Autodesk Inventor part; units mm, degrees
ref_plane "YZ Plane" through (0, 0, 0) normal (1, 0, 0) x (0, 1, 0)
ref_plane "XZ Plane" through (0, 0, 0) normal (0, 1, 0) x (-1, 0, 0)
ref_plane "XY Plane" through (0, 0, 0) normal (0, 0, 1) x (1, 0, 0)
sketch "Эскиз1" plane through (0, 0, 0) normal (0, 1, 0) x (-1, 0, 0)
  line L0 (0, -6.5) -> (-2.25, -6.5)
  line L1 (-2.25, -6.5) -> (-4.25, -6.5)
  line L2 (-2.25, -6.5) -> (-4.25, -6.5)
  line L3 (-6.5, -6.5) -> (-4.25, -6.5)
  line L4 (0, -6.5) -> (0, 0.5)
  line L5 (0, 0.5) -> (-6.5, 0.5)
  line L6 (-6.5, 0.5) -> (-6.5, -6.5)
  line L7 (-2.25, -6.5) -> (-2.25, -1.5)
  line L8 (-2.25, -1.5) -> (-4.25, -1.5)
  line L9 (-4.25, -1.5) -> (-4.25, -6.5)
  point P0 (0, 0)
  dimension "d2" = 2.25
  dimension "d4" = 2
  dimension "d31" = 7
  dimension "d32" = 5
extrude "Выдавливание1" add sketch "Эскиз1" along normal blind 21
sketch "Эскиз2" plane through (0, 21, 0) normal (0, 1, 0) x (1, 0, 0)
  line L0 (4.25, 2) -> (2.25, 2)
  line L1 (4.25, 6.5) -> (2.25, 6.5)
  line L2 (2.25, 6.5) -> (2.25, 2)
  line L3 (2.25, 2) -> (4.25, 2)
  line L4 (4.25, 2) -> (4.25, 6.5)
  point P0 (0, 0)
extrude "Выдавливание2" add sketch "Эскиз2" along normal blind 1.425 and the other way blind 22.425
sketch "Эскиз4" plane through (2.25, 0, -2) normal (0, 0, 1) x (1, 0, 0)
  line L0 (0, 22.425) -> (2, 22.425)
  line L1 (2, -1.425) -> (0, -1.425)
  line L2 (-2.25, 21) -> (4.75, 21)
  line L3 (-2.25, 0) -> (4.75, 0)
  line L4 (4.75, 0) -> (4.75, 21)
  line L5 (-2.25, 1) -> (-2.25, 20)
  line L6 (0, 22.425) -> (0, 21)
  line L7 (2, 21) -> (2, 22.425)
  dimension "d17" = 23.85
  dimension "d18" = 21
  dimension "d19" = 7
  dimension "d20" = 2.25
  dimension "d21" = 2
  dimension "d22" = 2.75
  dimension "d23" = 1.425
  dimension "d24" = 7
sketch "Эскиз6" plane through (0, 0, 0.5) normal (0, 0, 1) x (1, 0, 0)
  line L0 (0, 0) -> (0, 1.5)
  line L1 (0, 0) -> (0, 21)
  line L2 (0, 21) -> (6.5, 21)
  line L3 (0, 21) -> (0, 19.5)
  line L4 (0, 19.5) -> (5, 19.5)
  line L5 (5, 19.5) -> (5, 1.5)
  line L6 (5, 1.5) -> (0, 1.5)
  line L7 (0, 1.5) -> (0, 19.5)
  dimension "d33" = 1.5
  dimension "d34" = 1.5
  dimension "d35" = 5
extrude "Выдавливание5" cut sketch "Эскиз6" against normal blind 5
sketch "Эскиз7" plane through (6.5, 0, 0.5) normal (1, 0, 0) x (0, 0, -1)
  line L0 (7, 0) -> (7, 21)
  line L1 (7, 10.5) -> (7, 18)
  line L2 (7, 18) -> (7, 3)
  line L3 (0, 19.5) -> (0, 1.5)
  line L4 (0, 3) -> (7, 3)
  line L5 (0, 18) -> (7, 18)
  line L6 (7, 18) -> (4, 18)
  line L7 (4.5, 18) -> (4.5, 3)
  line L8 (4.5, 3) -> (2, 3)
  circle A0 centre (2, 3) radius 1.25
  circle A1 centre (4.25, 18) radius 1.25
  line L9 (5, 19.5) -> (5, 1.5)
  line L10 (5, 1.5) -> (5, 19.5)
  line L11 (5, 3) -> (5, 5)
  line L12 (5, 5) -> (5, 7)
  line L13 (5, 7) -> (5, 9)
  line L14 (5, 9) -> (5, 11)
  line L15 (5, 11) -> (5, 13)
  line L16 (5, 13) -> (5, 15)
  circle A2 centre (5, 5) radius 0.6
  circle A3 centre (5, 7) radius 0.6
  circle A4 centre (5, 9) radius 0.6
  circle A5 centre (5, 11) radius 0.6
  circle A6 centre (5, 13) radius 0.6
  circle A7 centre (5, 15) radius 0.6
  point P0 (0.5, 0)
  dimension "d38" = 7.5
  dimension "d39" = 15
  dimension "d40" = 3
  dimension "d41" = 0.5
  dimension "d42" = 2.5
  dimension "d43" = 2.5
  dimension "d44" = 2.5
  dimension "d61" = 2
  dimension "d62" = 2
  dimension "d63" = 2
  dimension "d64" = 2
  dimension "d65" = 2
  dimension "d66" = 2
  dimension "d68" = 1.2
  dimension "d69" = 1.2
  dimension "d70" = 1.2
  dimension "d71" = 1.2
  dimension "d72" = 1.2
  dimension "d73" = 1.2
extrude "Выдавливание6" add sketch "Эскиз7" along normal blind 1.7 contours A2 L7 L9 | L9 A2 | A1 L9 L5 | L5 L9 A1 | A0 L4 | L4 A0 | A2 L7 | L9 A1 L7 L5 | L5 A1 L9 | L7 A1 L5 | A7 L9 | L9 A7 L7 | A3 L7 | L7 A3 L9 | L9 A3 | L7 A7 | A4 L7 | L7 A4 L9 | A6 L9 L7 | L7 A6 | A6 L9 | L9 A4 | A5 L7 | L7 A5 L9 | L9 A5
properties part number "fast_battery"
The listing builds one solid part. Answer for the finished solid, in the listing's coordinates (mm). A direction names the side the tool comes from. Coordinates: 2 decimals unless noted, no trailing zeros. Loops run counter-clockwise (first coordinate to the right, second up) from the corner with the lowest first, then second, coordinate; pieces in that order, holes last. Notation, with made-up numbers: M 37,24.25 L 46,24.25 A21 ccw 46,56.25 Z; hole C 35.25,6.5 d5. An arc over 180 degrees is marked long. Answer as a JSON object with one key per item and string values. Group by question number.
Item 1: Consider L1, parallel to Y at x = 4, z = -3.5 (3 decimals); L2, parallel to Y at x = 1.5, z = -0.75; L3, parallel to X at y = 10.5, z = -3. Determine where each line is inside the solid, lowest interval first.
Item 2: Which of the six approach directions +Z, -Z, +X, -X, +Y, -Y give full straight-line access (tool end or side, diameter ignored) to faces 4 (the face through (3, -1, -2)), 5 (the face through (7.34, 14.59, -4.06)), 6 (the face through (4.25, 22, -4))?
Item 3: Each of these flat-tipped pins is pushed along its axis until it touches: P1, Ø1.1, axis at x = 3, y = 22, coming from the +Z side; P2, Ø1.5, axis at x = 6, z = -2, coming from the -Y side; P3, Ø0.7, axis at y = -1, z = -5, coming from the +X side. Where does it stop, or does it pass through?
Item 4: Determine the mould class of faces 1 (the face through (3, -1.425, -4)), 2 (the face through (7.338, 11.586, -4.37)), 3 (the face through (8.2, 9, -4.5)) for opening direction Y: +Y half, -Y half, draft (parallel to the pull), parting line (faces both ways), or undercut.
Item 5: Section C-C (z = -1.5) is taken. Write down the section's boundary in (x, y), and give its area (4 significant figures).
Item 6: Section B-B (y = 15) is taken. Write down the section's boundary in (x, z), and give its area (3 significant figures).
Item 7: Section D-D (y = 8) is taken. Write down the section's boundary in (x, z).
Item 8: Section A-A (x = 3.5) is taken. Write down the section's boundary in (y, z) (3 decimals), and give its area (3 significant figures).
Solved:
{
 "1": {"L1": "y = -1.425 to 1.5, 19.5 to 22.425", "L2": "y = 0 to 1.5, 19.5 to 21", "L3": "x = 5 to 6.5"},
 "2": {"face 4": "+Z, +X, -X, -Y", "face 5": "+X", "face 6": "+Z, -Z, +X, +Y"},
 "3": {"P1": "stops at z = -2", "P2": "stops at y = 0", "P3": "stops at x = 4.25"},
 "4": {"face 1": "-Y half", "face 2": "undercut", "face 3": "draft"},
 "5": {"outline": "M 0,0 L 6.5,0 L 6.5,1.75 L 8.2,1.75 L 8.2,4.25 L 6.5,4.25 L 6.5,21 L 0,21 L 0,19.5 L 5,19.5 L 5,1.5 L 0,1.5 Z", "area": "50.75 mm2"},
 "6": {"outline": "M 0,-6.5 L 6.5,-6.5 L 6.5,-5.1 L 8.2,-5.1 L 8.2,-3.9 L 6.5,-3.9 L 6.5,0.5 L 5,0.5 L 5,-4.5 L 0,-4.5 Z", "area": "22.5 mm2"},
 "7": {"outline": "M 0,-6.5 L 6.5,-6.5 L 6.5,0.5 L 5,0.5 L 5,-4.5 L 0,-4.5 Z"},
 "8": {"outline": "M -1.425,-6.5 L 22.425,-6.5 L 22.425,-2 L 21,-2 L 21,0.5 L 19.5,0.5 L 19.5,-4.5 L 1.5,-4.5 L 1.5,0.5 L 0,0.5 L 0,-2 L -1.425,-2 Z", "area": "69.8 mm2"}
}
